The drawing under review shows one solid part. Ordinate dimensions are in mm from its lowest x, y, z. A direction names the side the tool comes from. Coordinates: 2 decimals unless noted, no trailing zeros. Write each loop counter-clockwise with the first axis right and the second up, starting at its lowest first coordinate (ties: lowest second). Pieces come first, ordered by that corner, then holes.
Q1. Mouldability with a two-part tool opening along X and no side actions: class the marked faces 1, 2, 3 and 4 as pulls with the +X half, pulls with the -X half, needs draft (parallel to the pull), parting line crosses it, or undercut.
Q2. For probe 1 along Y at (x, z) = (2, 1); probe 2 along X at (y, z) = (28, 11); probe 3 along Y at (x, z) = (6.5, 6), list the stretches that pass through material, from the lowest coordinate up.
Q3. Insertion check: pin 1 (1.8 mm diameter, centred on x = 5, z = 5.5, fed in from -Y); pin 2 (3.5 mm diameter, centred on y = 11, z = 10, fed in from -X); pin 3 (4 mm diameter, centred on x = 24, z = 22, fed in from +Y); pin 4 (1.8 mm diameter, centred on x = 38, y = 2, fed in from +Z). Each pin has a flat end and moves straight along its axis. Give the tip position at first contact, or say it passes through.
Q4. Take a section at C-C (z = 11.5). Give the boundary of the cut face in (x, y).
Q5. Machinability: for the marked faces 5, 6, 7, 8 and 9, which of the approach directions +Z, -Z, +X, -X, +Y, -Y give a long, thin tool a straight path to every point of the face, cutting with its end or side? Answer none if there is none.
Q6. Take a section at A-A (y = 2). Give the boundary of the cut face in (x, z).
Q7. Take a section at B-B (x = 38). Give the boundary of the cut face in (y, z).
Q8. Take a section at D-D (y = 23). Give the boundary of the cut face in (x, z), and give its area (3 significant figures).
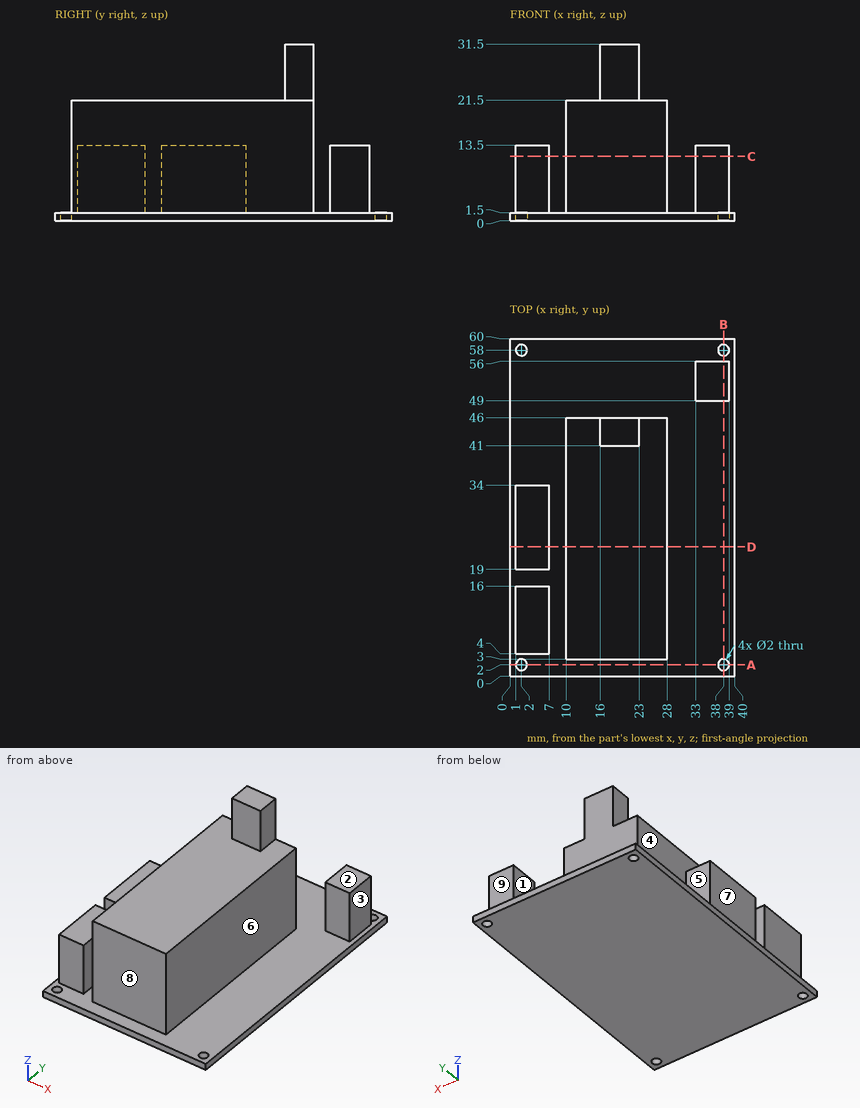
Response:
1. face 1: pulls with the -X half
1. face 2: needs draft
1. face 3: pulls with the +X half
1. face 4: undercut
2. probe 1: y = 0 to 1, 3 to 57, 59 to 60
2. probe 2: x = 1 to 7, 10 to 28
2. probe 3: y = 4 to 16, 19 to 34
3. pin 1: stops at y = 4
3. pin 2: stops at x = 1
3. pin 3: stops at y = 46
3. pin 4: passes through
4. outline: (1, 4) - (7, 4) - (7, 16) - (1, 16) - close; (1, 19) - (7, 19) - (7, 34) - (1, 34) - close; (10, 3) - (28, 3) - (28, 46) - (10, 46) - close; (33, 49) - (39, 49) - (39, 56) - (33, 56) - close
5. face 5: +Z, -X, +Y
5. face 6: +Z, +X, +Y, -Y
5. face 7: +Z, -X, +Y, -Y
5. face 8: +Z, +X, -X, -Y
5. face 9: +Z, +X, -X, +Y
6. outline: (0, 0) - (1, 0) - (1, 1.5) - (0, 1.5) - close; (3, 0) - (37, 0) - (37, 1.5) - (3, 1.5) - close; (39, 0) - (40, 0) - (40, 1.5) - (39, 1.5) - close
7. outline: (0, 0) - (1, 0) - (1, 1.5) - (0, 1.5) - close; (3, 0) - (57, 0) - (57, 1.5) - (56, 1.5) - (56, 13.5) - (49, 13.5) - (49, 1.5) - (3, 1.5) - close; (59, 0) - (60, 0) - (60, 1.5) - (59, 1.5) - close
8. outline: (0, 0) - (40, 0) - (40, 1.5) - (28, 1.5) - (28, 21.5) - (10, 21.5) - (10, 1.5) - (7, 1.5) - (7, 13.5) - (1, 13.5) - (1, 1.5) - (0, 1.5) - close
8. area: 492 mm2
